from build123d import *

# Parameters (mm, degrees)
SKETCH1_R           = 2.5
SKETCH1_R_2         = 12.5
BOSS_EXTRUDE1_DEPTH = 5
BOSS_EXTRUDE2_DEPTH = 5
FILLET1_R           = 5
SKETCH3_R           = 6
CUT_EXTRUDE1_DEPTH  = 10


with BuildPart() as part:
    # Sketch1 → Boss-Extrude1 (new body)
    with BuildSketch(Plane(origin=(0, 0, 0), x_dir=(1, 0, 0), z_dir=(0, 1, 0))):
        with BuildLine():
            Line((90, 60), (90, -60))
            Line((90, -60), (-9.08206944, -29.639770827))
            ThreePointArc((-9.08206944, -29.639770827), (-31, 0), (-9.08206944, 29.639770827))
            Line((-9.08206944, 29.639770827), (90, 60))
        make_face()
        with Locations(Location((0, 25.5, 0), (0, 0, 270))):
            Circle(SKETCH1_R, mode=Mode.SUBTRACT)
        with Locations(Location((-25.5, 0, 0), (0, 0, 270))):
            Circle(SKETCH1_R, mode=Mode.SUBTRACT)
        with Locations(Location((25.5, 0, 0), (0, 0, 270))):
            Circle(SKETCH1_R, mode=Mode.SUBTRACT)
        with Locations(Location((0, -25.5, 0), (0, 0, 270))):
            Circle(SKETCH1_R, mode=Mode.SUBTRACT)
        with Locations(Location((0, 0, 0), (0, 0, 270))):
            Circle(SKETCH1_R_2, mode=Mode.SUBTRACT)
    extrude(amount=BOSS_EXTRUDE1_DEPTH)

    # Sketch2 → Boss-Extrude2 (add)
    with BuildSketch(Plane(origin=(90, 0, 0), x_dir=(0, 0, -1), z_dir=(1, 0, 0))):
        with BuildLine():
            Line((-60, 0), (60, 0))
            Line((60, 0), (60, 30))
            ThreePointArc((60, 30), (57.071067812, 37.071067812), (50, 40))
            Line((50, 40), (-50, 40))
            ThreePointArc((-50, 40), (-57.071067812, 37.071067812), (-60, 30))
            Line((-60, 30), (-60, 0))
        make_face()
    extrude(amount=BOSS_EXTRUDE2_DEPTH)

    # Fillet1
    fillet1_edges = [part.edges().sort_by_distance(p)[0] for p in [
        (95, 0, 0),
        (90, 5, 0),
    ]]
    fillet(fillet1_edges, radius=FILLET1_R)

    # Sketch3 → Cut-Extrude1 (cut)
    with BuildSketch(Plane(origin=(95, 0, 0), x_dir=(0, 0, -1), z_dir=(1, 0, 0))):
        with Locations((-40, 22)):
            Circle(SKETCH3_R)
        with Locations((40, 22)):
            Circle(SKETCH3_R)
    extrude(amount=-CUT_EXTRUDE1_DEPTH, mode=Mode.SUBTRACT)


solid = part.part
Design review of the part built by this model. Coordinates are the model's own, in mm. A direction names the side the tool comes from. Round coordinates to 2 decimals unless told otherwise and drop trailing zeros. Order: outer loops, then holes, each group sorted by start corner. A loop starts at its lowest first (then second) coordinate and runs counter-clockwise, first axis right, second up.
1) Consider section A-A (z = 0). State the section outline as (x, y) points, plus the area to 3 significant figures.
The answers:
outline: (-31, 0) - (-28, 0) - (-28, 5) - (-31, 5) - close; (-23, 0) - (-12.5, 0) - (-12.5, 5) - (-23, 5) - close; (12.5, 0) - (23, 0) - (23, 5) - (12.5, 5) - close; (28, 0) - (90, 0) arc R5 ccw to (95, 5) - (95, 40) - (90, 40) - (90, 10) arc R5 cw to (85, 5) - (28, 5) - close
area: 630 mm2
2) For L1, parallel to X at y = 2, z = 0; L2, parallel to X at y = 1.6, z = 0; L3, parallel to Y at x = -19.5, z = -16, list the stretches that pass through material, from the lowest coordinate up.
The answers:
L1: x = -31 to -28, -23 to -12.5, 12.5 to 23, 28 to 94
L2: x = -31 to -28, -23 to -12.5, 12.5 to 23, 28 to 93.67
L3: y = 0 to 5
3) Consider section C-C (y = 25). State the section outline as (x, z) points, plus the area to 3 significant figures.
The answers:
outline: (90, -60) - (95, -60) - (95, -45.2) - (90, -45.2) - close; (90, -34.8) - (95, -34.8) - (95, 34.8) - (90, 34.8) - close; (90, 45.2) - (95, 45.2) - (95, 60) - (90, 60) - close
area: 496 mm2
4) Consider section D-D (z = 40). State the section outline as (x, y) points.
The answers:
outline: (24.73, 0) - (90, 0) arc R5 ccw to (95, 5) - (95, 16) - (90, 16) - (90, 10) arc R5 cw to (85, 5) - (24.73, 5) - close; (90, 28) - (95, 28) - (95, 40) - (90, 40) - close
5) Clearance check with flat-ended pins moving along their axes: pin 1 Ø10 at (y, z) = (25, 16) entering from -X; pin 2 Ø1.5 at (x, z) = (78, -46.5) entering from +Y. State where each tip first meets the part, or that it passes through.
The answers:
pin 1: stops at x = 90
pin 2: stops at y = 5
6) Draft analysis for pull direction Z (two halves, no side actions). For faces 3 (the flat face through (39.77, 2.71, -44.61)), 4 (the flat face through (42, 0, 1)), 5 (the cylindrical face through (3.755, 2.465, 11.923)), state which applies: released by +Z, released by -Z, zero draft, split by the parting line, or undercut.
The answers:
face 3: released by -Z
face 4: zero draft
face 5: undercut
7) Consider section B-B (x = 0). State the section outline as (y, z) points, plus the area to 3 significant figures.
The answers:
outline: (0, -32.42) - (5, -32.42) - (5, -28) - (0, -28) - close; (0, -23) - (5, -23) - (5, -12.5) - (0, -12.5) - close; (0, 12.5) - (5, 12.5) - (5, 23) - (0, 23) - close; (0, 28) - (5, 28) - (5, 32.42) - (0, 32.42) - close
area: 149 mm2
8) Machinability: for faces 1 (the flat face through (41, 5, -1)), 2 (the cylindrical face through (0, 2, 23)), which of the approach directions +Z, -Z, +X, -X, +Y, -Y give a long, thin tool a straight path to every point of the face, cutting with its end or side? Answer none if there is none.
The answers:
face 1: +Z, -Z, -X, +Y
face 2: +Y, -Y
